```python
from build123d import *

# Parameters (mm, degrees)
F0_W      = 499
F0_H      = 500
F1_DEPTH  = 179
F2_T      = -5
F3_W      = 493
F3_H      = 493
F4_DEPTH  = 10
F5_W      = 149
F5_H      = 109
F6_DEPTH  = 4.5
F7_W      = 136
F7_H      = 96
F8_DEPTH  = 60.5
F9_R      = 11.15
F10_DEPTH = 25
F11_R     = 8
F11_R_2   = 4.5
F12_DEPTH = 25
F13_R     = 4
F14_DEPTH = 10


with BuildPart() as f1:
    # F0 (on Top) → F1 (new body)
    with BuildSketch(Plane.XY):
        Rectangle(F0_W, F0_H)
    extrude(amount=-F1_DEPTH)

    # F2
    f2_openings = [f1.faces().sort_by_distance(p)[0] for p in [
        (0, 0, 0),
    ]]
    offset(amount=F2_T, openings=f2_openings)

    # F3 (on Top) → F4 (join)
    with BuildSketch(Plane.XY):
        Rectangle(F3_W, F3_H)
    extrude(amount=F4_DEPTH)

    # F5 (on face) → F6 (join)
    with BuildSketch(Plane.XY.offset(10)):
        with Locations((-112, 132)):
            Rectangle(F5_W, F5_H)
    extrude(amount=F6_DEPTH)

    # F7 (on face) → F8 (cut)
    with BuildSketch(Plane.XY.offset(14.5)):
        with Locations((-112, 132)):
            Rectangle(F7_W, F7_H)
    extrude(amount=-F8_DEPTH, mode=Mode.SUBTRACT)

    # F9 (on face) → F10 (cut)
    with BuildSketch(Plane.XY.offset(10)):
        with Locations((-76.5, 26.5)):
            Circle(F9_R)
        with Locations((-161.5, 26.5)):
            Circle(F9_R)
    extrude(amount=-F10_DEPTH, mode=Mode.SUBTRACT)

    # F11 (on face) → F12 (cut)
    with BuildSketch(Plane(origin=(0, 0, -179), x_dir=(1, 0, 0), z_dir=(0, 0, -1))):
        with Locations((-150.940314, 223.095)):
            Circle(F11_R)
        with Locations((0, 160.243019)):
            Circle(F11_R_2)
        with Locations((0, 225.243019)):
            Circle(F11_R_2)
    extrude(amount=-F12_DEPTH, mode=Mode.SUBTRACT)

    # F13 (on face) → F14 (cut)
    with BuildSketch(Plane.XZ.offset(250)):
        with Locations((-226, -23.5)):
            Circle(F13_R)
        with Locations((-226, -155.5)):
            Circle(F13_R)
        with Locations((226, -155.5)):
            Circle(F13_R)
        with Locations((226, -23.5)):
            Circle(F13_R)
    extrude(amount=-F14_DEPTH, mode=Mode.SUBTRACT)


solid = f1.part
```
Part model, mm, in its own coordinate system. A direction names the side the tool comes from. Round coordinates to 2 decimals unless told otherwise and drop trailing zeros. Write each loop counter-clockwise with the first axis right and the second up, starting at its lowest first coordinate (ties: lowest second). Pieces come first, ordered by that corner, then holes. Notation, with made-up numbers: (9, -17) -> (21, -17) arc R11 cw to (21, -9) -> close; hole circle Ø2 at (47, 37.25). An arc over 180 degrees is marked (long way). Return JSON: item names as keys, results as strings. Group by question number.
Q1. Saw through at B-B on y = -198. Write the cut outline in (x, z).
Q2. Saw through at C-C on x = -76.5. Write the cut outline in (y, z).
Q3. Saw through at D-D on z = -8. Write the cut outline in (x, y).
Q4. Saw through at A-A on y = 26.5. Write the cut outline in (x, z).
Q5. Pin check, flat tips, straight feed: pin 1 (5 mm diameter, centred on x = 29.5, z = 7, fed in from -Y); pin 2 (2 mm diameter, centred on x = 75, y = 21.5, fed in from +Z); pin 3 (5.5 mm diameter, centred on x = 0, y = -225.24, fed in from -Z). Stop position of each tip, or through.
Q6. Mould opens along Z. For faces 1 (the flat face through (-3, 4, -179)), 2 (the flat face through (-3, -245, -86)), 3 (the flat face through (-3, 250, -88)) say: pulls with the +Z half, pulls with the -Z half, needs draft (parallel to the pull), parting line crosses it, or undercut.
Q7. Which spindle directions (+Z, -Z, +X, -X, +Y, -Y) get a long thin tool onto all of the face, cutting with end or side? Do faces 4 (the cylindrical face through (-157.29, -218.23, -176.54)), 5 (the flat face through (-249.5, -3, -88)), 6 (the flat face through (-180, 131, 7)), 7 (the flat face through (-3, 245, -86)). Say none if no direction does.
Q8. Probe L1, parallel to Y at x = 0, z = -175.4; L2, parallel to Y at x = -76.5, z = 3.5; L3, parallel to Z at x = -226, y = -246.2. List the from-to ranges inside material, lowest first. Write a range as [from, to].
Answer:
{
 "1": {"outline": "(-249.5, -179) -> (249.5, -179) -> (249.5, 0) -> (246.5, 0) -> (246.5, 10) -> (-246.5, 10) -> (-246.5, 0) -> (-249.5, 0) -> close; hole (-244.5, -174) -> (244.5, -174) -> (244.5, 0) -> (-244.5, 0) -> close"},
 "2": {"outline": "(-250, -179) -> (250, -179) -> (250, 0) -> (246.5, 0) -> (246.5, 10) -> (186.5, 10) -> (186.5, 14.5) -> (180, 14.5) -> (180, 0) -> (245, 0) -> (245, -174) -> (-245, -174) -> (-245, 0) -> (15.35, 0) -> (15.35, 10) -> (-246.5, 10) -> (-246.5, 0) -> (-250, 0) -> close; (37.65, 0) -> (84, 0) -> (84, 14.5) -> (77.5, 14.5) -> (77.5, 10) -> (37.65, 10) -> close"},
 "3": {"outline": "(-249.5, -250) -> (249.5, -250) -> (249.5, 250) -> (-249.5, 250) -> close; hole (-244.5, -245) -> (244.5, -245) -> (244.5, 245) -> (-244.5, 245) -> close"},
 "4": {"outline": "(-249.5, -179) -> (249.5, -179) -> (249.5, 0) -> (246.5, 0) -> (246.5, 10) -> (-65.35, 10) -> (-65.35, 0) -> (244.5, 0) -> (244.5, -174) -> (-244.5, -174) -> (-244.5, 0) -> (-172.65, 0) -> (-172.65, 10) -> (-246.5, 10) -> (-246.5, 0) -> (-249.5, 0) -> close; (-150.35, 0) -> (-87.65, 0) -> (-87.65, 10) -> (-150.35, 10) -> close"},
 "5": {"pin 1": "y = -246.5", "pin 2": "z = 10", "pin 3": "z = 0"},
 "6": {"face 1": "pulls with the -Z half", "face 2": "undercut", "face 3": "needs draft"},
 "7": {"face 4": "-Z", "face 5": "+Z, -Z, -X, +Y, -Y", "face 6": "+Z", "face 7": "none"},
 "8": {"L1": "[-250, -229.74], [-220.74, -164.74], [-155.74, 250]", "L2": "[-246.5, 15.35], [37.65, 84], [180, 246.5]", "L3": "[-179, -159.5], [-151.5, -27.5], [-19.5, 10]"}
}
